Autodesk Inventor part; units mm, degrees
ref_plane "YZ Plane" through (0, 0, 0) normal (1, 0, 0) x (0, 1, 0)
ref_plane "XZ Plane" through (0, 0, 0) normal (0, 1, 0) x (-1, 0, 0)
ref_plane "XY Plane" through (0, 0, 0) normal (0, 0, 1) x (1, 0, 0)
sketch "Sketch1" plane through (0, 0, 0) normal (0, 1, 0) x (-1, 0, 0)
  line L0 (0, 0) -> (38.1, 0)
  line L1 (38.1, -25.4) -> (0, -25.4)
  line L2 (0, -25.4) -> (0, 0)
  line L3 (38.1, 0) -> (38.1, -25.4)
extrude "Extrusion1" add sketch "Sketch1" along normal blind 25.4
sketch "Sketch2" plane through (0, 0, 0) normal (1, 0, 0) x (0, 0, -1)
  point P0 (0, 0)
sketch "Sketch3" plane through (0, 0, 0) normal (1, 0, 0) x (0, 0, -1)
  line L0 (25.4, 0) -> (0, 0)
  line L1 (25.4, 0) -> (25.4, 25.4)
  line L2 (0, 25.4) -> (25.4, 25.4)
  line L3 (0, 0) -> (0, 25.4)
  line L4 (22.225, 3.175) -> (3.175, 3.175)
  line L5 (3.175, 3.175) -> (3.175, 22.225)
  line L6 (3.175, 22.225) -> (22.225, 22.225)
  line L7 (22.225, 22.225) -> (25.4, 22.225)
  line L8 (25.4, 0) -> (25.4, 25.4)
  line L9 (22.225, 3.175) -> (25.4, 3.175)
  line L10 (25.4, 22.225) -> (25.4, 3.175)
  dimension "d4" = 3.175
sketch "Sketch4" plane through (0, 25.4, 0) normal (0, 1, 0) x (1, 0, 0)
  line L0 (-63.5, 0) -> (-63.5, 25.4) construction
  line L1 (-63.5, 12.7) -> (0, 12.7) construction
  line L2 (0, 12.7) -> (-12.7, 12.7) construction
  line L3 (-12.7, 12.7) -> (-31.75, 12.7) construction
  circle A0 centre (-31.75, 12.7) radius 2.5797
  circle A1 centre (-12.7, 12.7) radius 2.5797
  point P0 (0, 0)
  point P1 (-38.1, 0)
  point P2 (-38.1, 25.4)
  dimension "d7" = 12.7
  dimension "d8" = 19.05
  dimension "d9" = 5.1594
  dimension "d10" = 5.1594
extrude "Extrusion3" cut sketch "Sketch4" against normal blind 63.5
extrude "Extrusion4" cut sketch "Sketch3" against normal blind 127 contours L9 L4 L5 L6 L7 L1
properties part number "wheel tip connector 1"
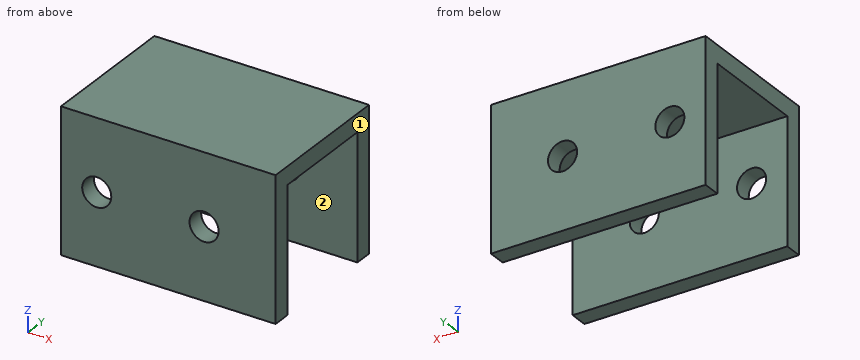
Could you check a few things on this model? Use its own coordinates, in mm. Face numbers are marked on the shaded views. A direction names the side the tool comes from. Coordinates: 2 decimals unless noted, no trailing zeros. Loops run counter-clockwise (first coordinate to the right, second up) from the corner with the lowest first, then second, coordinate; pieces in that order, holes last. Notation, with made-up numbers: M 77,7.5 L 102,7.5 A25 cw 102,20.5 Z; hole C 84.25,-10 d2. An arc over 180 degrees is marked long. Put each result on its own line as item: value. Start each with the question number.
(1) Suppose I cut it at C-C on y = 23.25. Please give me the cut outline in (x, z).
(2) Suppose I cut it at D-D on z = -12.7. Please give me the cut outline in (x, y) (3 decimals), then the cut area to 3 significant figures.
(3) Will these pins go through, and if not, where does the flat tip stop? P1, Ø6, axis at x = -31.75, z = -12.7, coming from the +Y side; P2, Ø1, axis at x = -13, z = -13, coming from the -Y side.
(4) Suppose I cut it at A-A on z = -22.25. Please give me the cut outline in (x, y) (3 decimals).
(5) Suppose I cut it at B-B on x = -12.7. Please give me the cut outline in (y, z) (3 decimals).
(6) For the marked faces 1 and 2, which set-ups out of +Z, -Z, +X, -X, +Y, -Y let a thin tool reach every point of the face, with its end or its side?
(7) I need wall thicknesses on line 1 (X direction, y = 0.85, z = -12.7); line 2 (Y direction, x = -16, z = -12.5) (3 decimals); line 3 (Z direction, x = -12.7, y = 22.9). Which ranges of each line are inside material? Lowest first, please. Write a range as from..to.
Solutions:
1. outline: M -38.1,-25.4 L 0,-25.4 L 0,0 L -38.1,0 Z; hole C -31.75,-12.7 d5.16; hole C -12.7,-12.7 d5.16
2. outline: M -38.1,0 L -34.33,0 L -34.33,3.175 L -38.1,3.175 Z; M -38.1,22.225 L -34.33,22.225 L -34.33,25.4 L -38.1,25.4 Z; M -29.17,0 L -15.28,0 L -15.28,3.175 L -29.17,3.175 Z; M -29.17,22.225 L -15.28,22.225 L -15.28,25.4 L -29.17,25.4 Z; M -10.12,0 L 0,0 L 0,3.175 L -10.12,3.175 Z; M -10.12,22.225 L 0,22.225 L 0,25.4 L -10.12,25.4 Z
2. area: 176 mm2
3. P1: stops at y = 25.4
3. P2: passes through
4. outline: M -38.1,0 L 0,0 L 0,3.175 L -38.1,3.175 Z; M -38.1,22.225 L 0,22.225 L 0,25.4 L -38.1,25.4 Z
5. outline: M 0,-25.4 L 3.175,-25.4 L 3.175,-15.28 L 0,-15.28 Z; M 0,-10.12 L 3.175,-10.12 L 3.175,-3.175 L 22.225,-3.175 L 22.225,-10.12 L 25.4,-10.12 L 25.4,0 L 0,0 Z; M 22.225,-25.4 L 25.4,-25.4 L 25.4,-15.28 L 22.225,-15.28 Z
6. face 1: +Z, -Z, +X, +Y, -Y
6. face 2: -Z, +X, -X
7. line 1: x = -38.1..-34.33, -29.17..-15.28, -10.12..0
7. line 2: y = 0..3.175, 22.225..25.4
7. line 3: z = -25.4..-15.28, -10.12..0
